The model under review builds one solid part; all positions refer to its coordinate system, in mm. A direction names the side the tool comes from. Round coordinates to 2 decimals unless told otherwise and drop trailing zeros. Order: outer loops, then holes, each group sorted by start corner. A loop starts at its lowest first (then second) coordinate and runs counter-clockwise, first axis right, second up. Notation, with made-up numbers: M 3.5,86 L 61.5,86 A22 ccw 61.5,103 Z; hole C -22,48.25 d11. An arc over 180 degrees is marked long. Answer as a JSON object with one key per item and string values. Group by question number.
1. Machinability: for faces 1 (the face through (530, -55.649, 348)), 2 (the face through (480.112, -94, 348)), which of the approach directions +Z, -Z, +X, -X, +Y, -Y give a long, thin tool a straight path to every point of the face, cutting with its end or side? Answer none if there is none.
2. Add section A-A on x = 539. State the section outline as (y, z) points, and give its area (3 significant figures).
3. Add section B-B on z = 358. State the section outline as (x, y) points, and give its area (4 significant figures).
4. Clearance check with flat-ended pins moving along their axes: P1, Ø1, axis at x = 541, y = -118, coming from the +Z side; P2, Ø6, axis at y = -110.5, z = 345.5, coming from the +X side. State where each tip first meets the part, or that it passes through.
5. Add section C-C on y = -102. State the section outline as (x, z) points, and give its area (3 significant figures).
6. To check wall thickness, follow probe 1 along Z at (x, y) = (527, -121); probe 2 along X at (y, z) = (-116, 359); probe 3 along Y at (x, z) = (517.5, 349.5). State the ranges of each line that lie inside material, in increasing order. Write a range as [from, to].
Autodesk Inventor part; units mm, degrees
ref_plane "YZ Plane" through (0, 0, 0) normal (1, 0, 0) x (0, 1, 0)
ref_plane "XZ Plane" through (0, 0, 0) normal (0, 1, 0) x (-1, 0, 0)
ref_plane "XY Plane" through (0, 0, 0) normal (0, 0, 1) x (1, 0, 0)
ref_plane "Arbeitsebene1" through (575.6121, -61.149, 338.1375) normal (-1, 0, 0) x (0, -1, 0)
sketch "Skizze1" plane through (575.6121, -61.149, 338.1375) normal (-1, 0, 0) x (0, -1, 0)
  line L0 (74, -2) -> (75, -1)
  line L1 (74, 0) -> (74, -2)
  line L2 (75, -3) -> (-7.5, -3)
  line L3 (-7.5, -3) -> (-7.5, 23)
  line L4 (-4.5, 22) -> (-3.5, 23)
  line L5 (-6.5, 22) -> (-4.5, 22)
  line L6 (-5.5, 23) -> (-6.5, 22)
  line L7 (-5.5, 23) -> (-7.5, 23)
  line L8 (75, -3) -> (75, -1)
  line L9 (74, -1) -> (-5.5, -1)
  line L10 (-5.5, -1) -> (-5.5, 22)
  point P0 (-61.149, -338.1375)
extrude "Extrusion1" add sketch "Skizze1" along normal blind 92.5
sketch "Skizze3" plane through (483.1121, -61.149, 338.1375) normal (-1, 0, 0) x (0, 0, 1)
  line L0 (-3, 7.5) -> (23, 7.5)
  line L1 (-3, -75) -> (23, -75)
  line L2 (23, -75) -> (23, 7.5)
  line L3 (23, 7.5) -> (-3, 7.5)
  line L4 (-3, 7.5) -> (-3, -75)
  point P0 (-338.1375, 61.149)
extrude "Extrusion2" add sketch "Skizze3" along normal blind 3
properties part number "BatCap"
Recorded:
{
 "1": {"face 1": "+Z, +X, -Y", "face 2": "+Z, -Z, -X, +Y, -Y"},
 "2": {"outline": "M -136.15,335.14 L -53.65,335.14 L -53.65,361.14 L -55.65,361.14 L -54.65,360.14 L -55.65,360.14 L -55.65,337.14 L -135.15,337.14 L -135.15,336.14 L -136.15,337.14 Z", "area": "212 mm²"},
 "3": {"outline": "M 480.11,-136.15 L 483.11,-136.15 L 483.11,-55.65 L 575.61,-55.65 L 575.61,-53.65 L 480.11,-53.65 Z", "area": "432.5 mm²"},
 "4": {"P1": "stops at z = 337.14", "P2": "stops at x = 483.11"},
 "5": {"outline": "M 480.11,335.14 L 575.61,335.14 L 575.61,337.14 L 483.11,337.14 L 483.11,361.14 L 480.11,361.14 Z", "area": "263 mm²"},
 "6": {"probe 1": "z = [335.14, 337.14]", "probe 2": "x = [480.11, 483.11]", "probe 3": "y = [-55.65, -53.65]"}
}
